For this review, take the finished solid that the model builds, in its own axes (mm). A direction names the side the tool comes from. Coordinates: 2 decimals unless noted, no trailing zeros. Loops run counter-clockwise (first coordinate to the right, second up) from the corner with the lowest first, then second, coordinate; pieces in that order, holes last. Notation, with made-up numbers: M 22.5,-16.5 L 34.5,-16.5 A22 ccw 34.5,-8.5 Z; hole C 46,14 d6. An arc over 180 degrees is marked long. Put each result on its own line as item: value.
```python
from build123d import *

# Parameters (mm, degrees)
SKETCH1_W           = 28
SKETCH1_H           = 48.18
SKETCH1_R           = 0.75
BOSS_EXTRUDE1_DEPTH = 1.59
SKETCH2_W           = 28
SKETCH2_H           = 1.59
BOSS_EXTRUDE2_DEPTH = 18
BOSS_EXTRUDE3_DEPTH = 1.59
BOSS_EXTRUDE4_START = -1.59
BOSS_EXTRUDE4_DEPTH = 1.59
SKETCH5_R           = 1.25
CUT_EXTRUDE1_DEPTH  = 6
SKETCH6_R           = 0.75
CUT_EXTRUDE2_DEPTH  = 6


with BuildPart() as part:
    # Sketch1 → Boss-Extrude1 (new body)
    with BuildSketch(Plane(origin=(0, 0, 0), x_dir=(1, 0, 0), z_dir=(0, 1, 0))):
        Rectangle(SKETCH1_W, SKETCH1_H)
        with Locations(Location((0, 7.5, 0), (0, 0, 90))):
            Circle(SKETCH1_R, mode=Mode.SUBTRACT)
        with Locations(Location((0, -7.5, 0), (0, 0, 90))):
            Circle(SKETCH1_R, mode=Mode.SUBTRACT)
        with Locations(Location((7.5, 0, 0), (0, 0, 90))):
            Circle(SKETCH1_R, mode=Mode.SUBTRACT)
        with Locations(Location((-7.5, 0, 0), (0, 0, 90))):
            Circle(SKETCH1_R, mode=Mode.SUBTRACT)
    extrude(amount=BOSS_EXTRUDE1_DEPTH)

    # Sketch2 → Boss-Extrude2 (add)
    with BuildSketch(Plane(origin=(0, 1.59, 0), x_dir=(1, 0, 0), z_dir=(0, 1, 0))):
        with Locations((0, 23.295)):
            Rectangle(SKETCH2_W, SKETCH2_H)
        with Locations((0, -23.295)):
            Rectangle(SKETCH2_W, SKETCH2_H)
    extrude(amount=BOSS_EXTRUDE2_DEPTH)

    # Sketch3 → Boss-Extrude3 (add)
    with BuildSketch(Plane.XY.offset(24.09)):
        with BuildLine():
            Line((-14, 19.59), (14, 19.59))
            ThreePointArc((14, 19.59), (0, 33.59), (-14, 19.59))
        make_face()
    extrude(amount=-BOSS_EXTRUDE3_DEPTH)

    # Sketch4 → Boss-Extrude4 (add)
    with BuildSketch(Plane(origin=(0, 0, -24.09), x_dir=(-1, 0, 0), z_dir=(0, 0, -1)).offset(BOSS_EXTRUDE4_START)):
        with BuildLine():
            Line((-14, 19.59), (14, 19.59))
            ThreePointArc((14, 19.59), (0, 33.59), (-14, 19.59))
        make_face()
    extrude(amount=BOSS_EXTRUDE4_DEPTH)

    # Sketch5 → Cut-Extrude1 (cut)
    with BuildSketch(Plane.XY.offset(24.09)):
        with Locations((0, 21)):
            Circle(SKETCH5_R)
    extrude(amount=-CUT_EXTRUDE1_DEPTH, mode=Mode.SUBTRACT)

    # Sketch6 → Cut-Extrude2 (cut)
    with BuildSketch(Plane(origin=(0, 0, -24.09), x_dir=(-1, 0, 0), z_dir=(0, 0, -1))):
        with Locations((0, 30.5)):
            Circle(SKETCH6_R)
        with Locations((0, 15.5)):
            Circle(SKETCH6_R)
        with Locations((7.5, 23)):
            Circle(SKETCH6_R)
        with Locations((-7.5, 23)):
            Circle(SKETCH6_R)
    extrude(amount=-CUT_EXTRUDE2_DEPTH, mode=Mode.SUBTRACT)


solid = part.part
```
(1) Add section D-D (y = 21). Write out the cut boundary in (x, z).
Determined:
outline: M -13.93,-24.09 L 13.93,-24.09 L 13.93,-22.5 L -13.93,-22.5 Z; M -13.93,22.5 L -1.25,22.5 L -1.25,24.09 L -13.93,24.09 Z; M 1.25,22.5 L 13.93,22.5 L 13.93,24.09 L 1.25,24.09 Z
(2) Add section B-B (z = 0). Write out the cut boundary in (x, y), plus the area to 4 significant figures.
Determined:
outline: M -14,0 L -8.25,0 L -8.25,1.59 L -14,1.59 Z; M -6.75,0 L 6.75,0 L 6.75,1.59 L -6.75,1.59 Z; M 8.25,0 L 14,0 L 14,1.59 L 8.25,1.59 Z
area: 39.75 mm^2
(3) Add section A-A (z = -7.5). Write out the cut boundary in (x, y).
Determined:
outline: M -14,0 L -0.75,0 L -0.75,1.59 L -14,1.59 Z; M 0.75,0 L 14,0 L 14,1.59 L 0.75,1.59 Z
(4) Wall thickness on line 1 along Z through (x, y) = (7.75, 19); line 2 along Y through (x, z) = (0, -23.3); line 3 along Y through (x, z) = (-9.25, 19.5): over which ranges is each line inside the solid? List them lowest first. Write a range as [from, to].
Determined:
line 1: z = [-24.09, -22.5], [22.5, 24.09]
line 2: y = [0, 14.75], [16.25, 29.75], [31.25, 33.59]
line 3: y = [0, 1.59]
(5) Draft analysis for pull direction Y (two halves, no side actions). For faces 1 (the cylindrical face through (0.098, 31.244, -23.306)), 2 (the flat face through (0, 17, 24.09)), 3 (the cylindrical face through (-0.308, 33.587, -23.284)), state which applies: +Y half, -Y half, draft (parallel to the pull), parting line (faces both ways), or undercut.
Determined:
face 1: undercut
face 2: draft
face 3: +Y half
(6) For pin 1 (2 mm diameter, centred on x = 0, z = 7.5, fed in from +Y); pin 2 (0.9 mm diameter, centred on x = 0, y = 15.5, fed in from -Z), all flat-tipped, find the tip position at first contact; note any pin that passes through.
Determined:
pin 1: stops at y = 1.59
pin 2: stops at z = 22.5
(7) Add section C-C (y = 8.5). Write out the cut boundary in (x, z), plus the area to 3 significant figures.
Determined:
outline: M -14,-24.09 L 14,-24.09 L 14,-22.5 L -14,-22.5 Z; M -14,22.5 L 14,22.5 L 14,24.09 L -14,24.09 Z
area: 89.0 mm^2
(8) Tool access review of faces 4 (the cylindrical face through (-0.03, 0.78, -6.75)), 5 (the cylindrical face through (-0.27, 19.78, 23.31)), 6 (the flat face through (0, 18, 22.5)), 7 (the cylindrical face through (-7.337, 22.268, -23.306)): name each direction out of +Z, -Z, +X, -X, +Y, -Y from which nothing blocks a thin tool from reaching the whole face with its end or side.
Determined:
face 4: +Y, -Y
face 5: +Z
face 6: +X, -X, +Y
face 7: -Z
